```python
from build123d import *

# Parameters (mm, degrees)
SKETCH_1_R               = 705
EXTRUDE_1_DEPTH          = 25
CUT_EXTRUDE_1_REACH      = 999.334
PATTERN_CIRCULAR_1_COUNT = 4
CUT_EXTRUDE_2_REACH      = 999.177
SKETCH_8_R               = 60
SKETCH_11_R              = 60
CUT_EXTRUDE_3_DEPTH      = 100
SKETCH_12_R              = 3
CUT_EXTRUDE_4_DEPTH      = 998.177266087
SKETCH_13_R              = 3
CUT_EXTRUDE_5_DEPTH      = 30


with BuildPart() as part:
    # 草图1 → 凸台-拉伸1 (new body)
    with BuildSketch(Plane(origin=(0, 0, 0), x_dir=(1, 0, 0), z_dir=(0, 1, 0))):
        with Locations(Location((0, 0, 0), (0, 0, 270))):
            Circle(SKETCH_1_R)
    extrude(amount=EXTRUDE_1_DEPTH)

    # 草图2 → 切除-拉伸1 (cut, up to next)
    with BuildSketch(Plane(origin=(0, 25, 0), x_dir=(1, 0, 0), z_dir=(0, 1, 0)), mode=Mode.PRIVATE) as cut_extrude_1_sk1:
        with BuildLine():
            Line((-12.5, -699.994189271), (-12.5, -704.889175687))
            ThreePointArc((-12.5, -704.889175687), (0, -705), (12.5, -704.889175687))
            Line((12.5, -704.889175687), (12.5, -699.994189271))
            Line((12.5, -699.994189271), (0, -678.343554177))
            Line((0, -678.343554177), (-12.5, -699.994189271))
        make_face()
    cut_extrude_1_tool1 = extrude(cut_extrude_1_sk1.sketch, amount=-CUT_EXTRUDE_1_REACH, mode=Mode.PRIVATE) & part.part
    cut_extrude_1 = cut_extrude_1_tool1.solids().sort_by_distance((0, 25, 695.82939))[0]
    add(cut_extrude_1, mode=Mode.SUBTRACT)

    # 阵列(圆周)1: 切除-拉伸1 ×4 about axis
    pattern_circular_1_axis = Axis((0, 0, 0), (0, 1, 0))
    for i in range(1, PATTERN_CIRCULAR_1_COUNT):
        add(cut_extrude_1.rotate(pattern_circular_1_axis, i * 360 / PATTERN_CIRCULAR_1_COUNT), mode=Mode.SUBTRACT)

    # 草图8 → 切除-拉伸2 (cut, up to next)
    with BuildSketch(Plane(origin=(0, 25, 0), x_dir=(1, 0, 0), z_dir=(0, 1, 0)), mode=Mode.PRIVATE) as cut_extrude_2_sk1:
        with Locations(Location((212.132034356, -212.132034356, 0), (0, 0, 270))):
            Circle(SKETCH_8_R)
    cut_extrude_2_tool1 = extrude(cut_extrude_2_sk1.sketch, amount=-CUT_EXTRUDE_2_REACH, mode=Mode.PRIVATE) & part.part
    # 草图8 → 切除-拉伸2 (cut, up to next)
    with BuildSketch(Plane(origin=(0, 25, 0), x_dir=(1, 0, 0), z_dir=(0, 1, 0)), mode=Mode.PRIVATE) as cut_extrude_2_sk2:
        with Locations(Location((-212.132034356, -212.132034356, 0), (0, 0, 270))):
            Circle(SKETCH_8_R)
    cut_extrude_2_tool2 = extrude(cut_extrude_2_sk2.sketch, amount=-CUT_EXTRUDE_2_REACH, mode=Mode.PRIVATE) & part.part
    # 草图8 → 切除-拉伸2 (cut, up to next)
    with BuildSketch(Plane(origin=(0, 25, 0), x_dir=(1, 0, 0), z_dir=(0, 1, 0)), mode=Mode.PRIVATE) as cut_extrude_2_sk3:
        with Locations(Location((-212.132034356, 212.132034356, 0), (0, 0, 270))):
            Circle(SKETCH_8_R)
    cut_extrude_2_tool3 = extrude(cut_extrude_2_sk3.sketch, amount=-CUT_EXTRUDE_2_REACH, mode=Mode.PRIVATE) & part.part
    # 草图8 → 切除-拉伸2 (cut, up to next)
    with BuildSketch(Plane(origin=(0, 25, 0), x_dir=(1, 0, 0), z_dir=(0, 1, 0)), mode=Mode.PRIVATE) as cut_extrude_2_sk4:
        with Locations(Location((212.132034356, 212.132034356, 0), (0, 0, 270))):
            Circle(SKETCH_8_R)
    cut_extrude_2_tool4 = extrude(cut_extrude_2_sk4.sketch, amount=-CUT_EXTRUDE_2_REACH, mode=Mode.PRIVATE) & part.part
    add(cut_extrude_2_tool1.solids().sort_by_distance((212.132034, 25, 212.132034))[0], mode=Mode.SUBTRACT)
    add(cut_extrude_2_tool2.solids().sort_by_distance((-212.132034, 25, 212.132034))[0], mode=Mode.SUBTRACT)
    add(cut_extrude_2_tool3.solids().sort_by_distance((-212.132034, 25, -212.132034))[0], mode=Mode.SUBTRACT)
    add(cut_extrude_2_tool4.solids().sort_by_distance((212.132034, 25, -212.132034))[0], mode=Mode.SUBTRACT)

    # 草图11 → 切除-拉伸3 (cut)
    with BuildSketch(Plane(origin=(0, 25, 0), x_dir=(1, 0, 0), z_dir=(0, 1, 0))):
        with Locations(Location((-73.369984345, -151.389388343, 0), (0, 0, 270))):
            Circle(SKETCH_11_R)
    extrude(amount=-CUT_EXTRUDE_3_DEPTH, mode=Mode.SUBTRACT)

    # 草图12 → 切除-拉伸4 (cut, through all)
    with BuildSketch(Plane.XZ):
        with Locations(Location((103.406710952, 73.607642412, 0), (0, 0, 270))):
            Circle(SKETCH_12_R)
        with Locations(Location((89.264575328, 59.465506788, 0), (0, 0, 270))):
            Circle(SKETCH_12_R)
    extrude(amount=-CUT_EXTRUDE_4_DEPTH, mode=Mode.SUBTRACT)

    # 草图13 → 切除-拉伸5 (cut)
    with BuildSketch(Plane.XZ):
        with Locations(Location((-76.905518251, 253.919871615, 0), (0, 0, 270))):
            Circle(SKETCH_13_R)
        with Locations(Location((-91.047653874, 239.777735991, 0), (0, 0, 90))):
            Circle(SKETCH_13_R)
    extrude(amount=-CUT_EXTRUDE_5_DEPTH, mode=Mode.SUBTRACT)


solid = part.part
```
Verification items for the finished model (mm, model axes). Give positions to 0.01 mm unless a question says otherwise; leave off trailing zeros. Order: outer loops, then holes, each group sorted by start corner. A loop starts at its lowest first (then second) coordinate and runs counter-clockwise, first axis right, second up. Notation, with made-up numbers: M 82.25,84 L 124.25,84 A20 cw 124.25,123 Z; hole C 34.5,-7.5 d6. An arc over 180 degrees is marked long. Return JSON: item names as keys, results as strings. Group by question number.
1) Mould release check, pull along X, two halves, no side actions. Record for faces 1 (the face through (-503.839, 12.325, 493.124)), 2 (the face through (10, 0, -10)), 3 (the face through (-96.35, 12.675, 206.814)): pulls with the +X half, pulls with the -X half, needs draft (parallel to the pull), parting line crosses it, or undercut.
2) Section check D-D on x = 169. Record the cut outline in (y, z).
3) Section check C-C on z = 187. Record the cut outline in (x, y).
4) Scan lines: line 1 (Z direction, x = 248, y = 3.25); line 2 (Z direction, x = 233.5, y = 11.5); line 3 (X direction, y = 14.5, z = 82.5). Record each from-to range of solid material in increasing order.
5) Section check A-A on y = 16.5. Give the number of separate pieces and of enclosed holes in the cut face, and give its area (3 significant figures).
6) Section check B-B on x = -190. Record the cut outline in (y, z), and give its area (3 significant figures).
7) Go/stop test with flat-tipped pins: pin 1 Ø5 at (x, y) = (-226.5, 10.5) entering from -Z; pin 2 Ø5 at (x, z) = (-91.05, 239.78) entering from +Y; pin 3 Ø1 at (x, y) = (-122.5, 14.5) entering from -Z; pin 4 Ø1.5 at (x, y) = (145, 20.5) entering from -Z. Record where each tip stops, or that it passes through.
Answer block:
{
 "1": {"face 1": "pulls with the -X half", "face 2": "needs draft", "face 3": "undercut"},
 "2": {"outline": "M 0,-684.44 L 25,-684.44 L 25,-253.84 L 0,-253.84 Z; M 0,-170.42 L 25,-170.42 L 25,170.42 L 0,170.42 Z; M 0,253.84 L 25,253.84 L 25,684.44 L 0,684.44 Z"},
 "3": {"outline": "M -679.75,0 L -266.61,0 L -266.61,25 L -679.75,25 Z; M -157.65,0 L -121.66,0 L -121.66,25 L -157.65,25 Z; M -25.08,0 L 157.65,0 L 157.65,25 L -25.08,25 Z; M 266.61,0 L 679.75,0 L 679.75,25 L 266.61,25 Z"},
 "4": {"line 1": "z = -659.94 to -260.23, -164.03 to 164.03, 260.23 to 659.94", "line 2": "z = -665.21 to -268.2, -156.07 to 156.07, 268.2 to 665.21", "line 3": "x = -700.16 to 700.16"},
 "5": {"separate pieces": "1", "enclosed holes": "9", "area": "1,500,000 mm^2"},
 "6": {"outline": "M 0,-678.91 L 25,-678.91 L 25,-267.9 L 0,-267.9 Z; M 0,-156.36 L 25,-156.36 L 25,156.36 L 0,156.36 Z; M 0,267.9 L 25,267.9 L 25,678.91 L 0,678.91 Z", "area": "28,400 mm^2"},
 "7": {"pin 1": "stops at z = -668.47", "pin 2": "passes through", "pin 3": "stops at z = -694.36", "pin 4": "stops at z = -690.08"}
}
